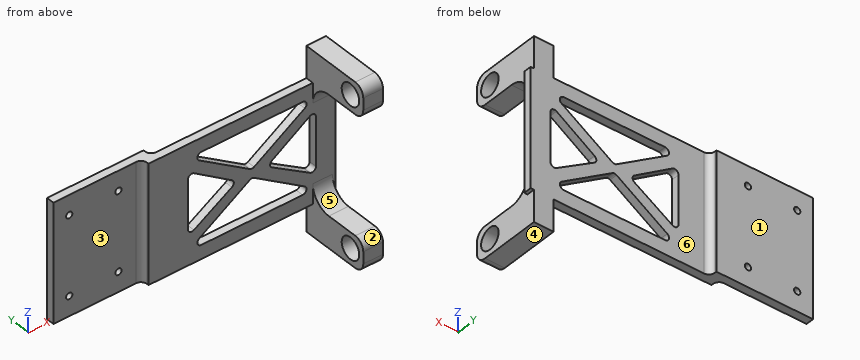
from build123d import *

# Parameters (mm, degrees)
BOSS_EXTRUDE1_DEPTH  = 60
FILLET1_R            = 3
CUT_EXTRUDE1_REACH   = 120.661
SKETCH2_R            = 1.6
CUT_EXTRUDE2_REACH   = 120.458
FILLET2_R            = 2
SKETCH5_W            = 10
SKETCH5_H            = 4
BOSS_EXTRUDE2_DEPTH  = 16
SKETCH6_W            = 10
SKETCH6_H            = 16
BOSS_EXTRUDE3_DEPTH  = 31.5
CUT_EXTRUDE3_REACH   = 163.612
SKETCH7_R            = 5.45
FILLET3_R            = 5
FILLET4_R            = 10
FILLET3_OF_MIRROR3_R = 5
FILLET4_OF_MIRROR3_R = 10


with BuildPart() as part:
    # Sketch1 → Boss-Extrude1 (new body)
    with BuildSketch(Plane.XY):
        Polygon((-37.939393939, 0.885392049), (7.060606061, 0.885392049), (7.060606061, -3.114607951), (102.060606061, -3.114607951), (102.060606061, 0.885392049), (11.060606061, 0.885392049), (11.060606061, 4.885392049), (-37.939393939, 4.885392049), align=None)
    extrude(amount=BOSS_EXTRUDE1_DEPTH)

    # Fillet1
    fillet1_edges = [part.edges().sort_by_distance(p)[0] for p in [
        (7.060606061, 0.885392049, 30),
        (11.060606061, 0.885392049, 30),
    ]]
    fillet(fillet1_edges, radius=FILLET1_R)

    # Sketch2 → Cut-Extrude1 (cut, up to next)
    with BuildSketch(Plane(origin=(0, 4.885392049, 0), x_dir=(1, 0, 0), z_dir=(0, 1, 0)), mode=Mode.PRIVATE) as cut_extrude1_sk1:
        with Locations(Location((-4.939393939, -50, 0), (0, 0, 180))):
            Circle(SKETCH2_R)
    cut_extrude1_tool1 = extrude(cut_extrude1_sk1.sketch, amount=-CUT_EXTRUDE1_REACH, mode=Mode.PRIVATE) & part.part
    # Sketch2 → Cut-Extrude1 (cut, up to next)
    with BuildSketch(Plane(origin=(0, 4.885392049, 0), x_dir=(1, 0, 0), z_dir=(0, 1, 0)), mode=Mode.PRIVATE) as cut_extrude1_sk2:
        with Locations(Location((-29.939393939, -50, 0), (0, 0, 180))):
            Circle(SKETCH2_R)
    cut_extrude1_tool2 = extrude(cut_extrude1_sk2.sketch, amount=-CUT_EXTRUDE1_REACH, mode=Mode.PRIVATE) & part.part
    cut_extrude1_1 = cut_extrude1_tool1.solids().sort_by_distance((-4.939394, 4.885392, 50))[0]
    add(cut_extrude1_1, mode=Mode.SUBTRACT)
    cut_extrude1_2 = cut_extrude1_tool2.solids().sort_by_distance((-29.939394, 4.885392, 50))[0]
    add(cut_extrude1_2, mode=Mode.SUBTRACT)
    cut_extrude1 = cut_extrude1_1 + cut_extrude1_2  # Cut-Extrude1 as one shape, for the pattern or mirror that repeats it

    # Mirror2: Cut-Extrude1 across plane
    add(cut_extrude1.mirror(Plane.XY.offset(30)), mode=Mode.SUBTRACT)

    # Sketch4 → Cut-Extrude2 (cut, up to next)
    with BuildSketch(Plane(origin=(0, 0.885392049, 0), x_dir=(1, 0, 0), z_dir=(0, 1, 0)), mode=Mode.PRIVATE) as cut_extrude2_sk1:
        Polygon((27.060606061, -14.276205352), (27.060606061, -46.276205352), (52.060606061, -29.743980797), align=None)
    cut_extrude2_tool1 = extrude(cut_extrude2_sk1.sketch, amount=-CUT_EXTRUDE2_REACH, mode=Mode.PRIVATE) & part.part
    # Sketch4 → Cut-Extrude2 (cut, up to next)
    with BuildSketch(Plane(origin=(0, 0.885392049, 0), x_dir=(1, 0, 0), z_dir=(0, 1, 0)), mode=Mode.PRIVATE) as cut_extrude2_sk2:
        Polygon((59.560606061, -32), (27.060606061, -53), (92.060606061, -53), align=None)
    cut_extrude2_tool2 = extrude(cut_extrude2_sk2.sketch, amount=-CUT_EXTRUDE2_REACH, mode=Mode.PRIVATE) & part.part
    # Sketch4 → Cut-Extrude2 (cut, up to next)
    with BuildSketch(Plane(origin=(0, 0.885392049, 0), x_dir=(1, 0, 0), z_dir=(0, 1, 0)), mode=Mode.PRIVATE) as cut_extrude2_sk3:
        Polygon((67.060606061, -29.743980797), (92.060606061, -14.276205352), (92.060606061, -46.276205352), align=None)
    cut_extrude2_tool3 = extrude(cut_extrude2_sk3.sketch, amount=-CUT_EXTRUDE2_REACH, mode=Mode.PRIVATE) & part.part
    # Sketch4 → Cut-Extrude2 (cut, up to next)
    with BuildSketch(Plane(origin=(0, 0.885392049, 0), x_dir=(1, 0, 0), z_dir=(0, 1, 0)), mode=Mode.PRIVATE) as cut_extrude2_sk4:
        Polygon((92.060606061, -7), (59.560606061, -28), (27.060606061, -7), align=None)
    cut_extrude2_tool4 = extrude(cut_extrude2_sk4.sketch, amount=-CUT_EXTRUDE2_REACH, mode=Mode.PRIVATE) & part.part
    add(cut_extrude2_tool1.solids().sort_by_distance((35.393939, 0.885392, 30.098797))[0], mode=Mode.SUBTRACT)
    add(cut_extrude2_tool2.solids().sort_by_distance((59.560606, 0.885392, 46))[0], mode=Mode.SUBTRACT)
    add(cut_extrude2_tool3.solids().sort_by_distance((83.727273, 0.885392, 30.098797))[0], mode=Mode.SUBTRACT)
    add(cut_extrude2_tool4.solids().sort_by_distance((59.560606, 0.885392, 14))[0], mode=Mode.SUBTRACT)

    # Fillet2
    fillet2_edges = [part.edges().sort_by_distance(p)[0] for p in [
        (59.560606061, -1.114607951, 32),
        (92.060606061, -1.114607951, 53),
        (27.060606061, -1.114607951, 53),
        (92.060606061, -1.114607951, 46.276205352),
        (67.060606061, -1.114607951, 29.743980797),
        (92.060606061, -1.114607951, 14.276205352),
        (27.060606061, -1.114607951, 7),
        (92.060606061, -1.114607951, 7),
        (59.560606061, -1.114607951, 28),
        (27.060606061, -1.114607951, 14.276205352),
        (52.060606061, -1.114607951, 29.743980797),
        (27.060606061, -1.114607951, 46.276205352),
    ]]
    fillet(fillet2_edges, radius=FILLET2_R)

    # Sketch5 → Boss-Extrude2 (add)
    with BuildSketch(Plane.XY.offset(60)):
        with Locations((95.422932692, -1.114607951)):
            Rectangle(SKETCH5_W, SKETCH5_H)
    boss_extrude2 = extrude(amount=BOSS_EXTRUDE2_DEPTH)

    # Sketch6 → Boss-Extrude3 (add)
    with BuildSketch(Plane.XZ.offset(3.114607951)):
        with Locations((95.422932692, 68)):
            Rectangle(SKETCH6_W, SKETCH6_H)
    boss_extrude3 = extrude(amount=BOSS_EXTRUDE3_DEPTH)

    # Sketch7 → Cut-Extrude3 (cut, up to next)
    with BuildSketch(Plane(origin=(100.422932692, 0, 0), x_dir=(0, 0, -1), z_dir=(1, 0, 0)), mode=Mode.PRIVATE) as cut_extrude3_sk1:
        with Locations((-68, -26.614607951)):
            Circle(SKETCH7_R)
    cut_extrude3_tool1 = extrude(cut_extrude3_sk1.sketch, amount=-CUT_EXTRUDE3_REACH, mode=Mode.PRIVATE) & part.part
    cut_extrude3 = cut_extrude3_tool1.solids().sort_by_distance((100.422933, -26.614608, 68))[0]
    add(cut_extrude3, mode=Mode.SUBTRACT)

    # Fillet3
    fillet3_edges = [part.edges().sort_by_distance(p)[0] for p in [
        (95.422932692, -34.614607951, 60),
        (95.422932692, -34.614607951, 76),
    ]]
    fillet(fillet3_edges, radius=FILLET3_R)

    # Fillet4
    fillet4_edges = [part.edges().sort_by_distance(p)[0] for p in [
        (95.422932692, -3.114607951, 60),
    ]]
    fillet(fillet4_edges, radius=FILLET4_R)

    # Mirror3: Boss-Extrude2, Boss-Extrude3, Cut-Extrude3 across plane
    add(boss_extrude2.mirror(Plane.XY.offset(30)))
    add(boss_extrude3.mirror(Plane.XY.offset(30)))
    add(cut_extrude3.mirror(Plane.XY.offset(30)), mode=Mode.SUBTRACT)

    # Fillet3 of Mirror3
    fillet3_of_mirror3_edges = [part.edges().sort_by_distance(p)[0] for p in [
        (95.422932692, -34.614607951, 0),
        (95.422932692, -34.614607951, -16),
    ]]
    fillet(fillet3_of_mirror3_edges, radius=FILLET3_OF_MIRROR3_R)

    # Fillet4 of Mirror3
    fillet4_of_mirror3_edges = [part.edges().sort_by_distance(p)[0] for p in [
        (95.422932692, -3.114607951, 0),
    ]]
    fillet(fillet4_of_mirror3_edges, radius=FILLET4_OF_MIRROR3_R)


solid = part.part
Geometry: final body of the model. Coordinates: model frame, mm. Face numbers are marked on the shaded views. A direction names the side the tool comes from. Round coordinates to 2 decimals unless told otherwise and drop trailing zeros. Order: outer loops, then holes, each group sorted by start corner. A loop starts at its lowest first (then second) coordinate and runs counter-clockwise, first axis right, second up. Notation, with made-up numbers: (-38.5, 71.5) -> (-34.5, 71.5) arc R28 cw to (-34.5, 97.5) -> close; hole circle Ø6 at (-15.5, 70). An arc over 180 degrees is marked (long way). Put each result on its own line as item: value. Start each with the question number.
Q1. Pull-direction query (Z, two-part tool) for the marked faces 4, 5 and 6; classes: +Z half, -Z half, draft (parallel to the pull), parting line (faces both ways), or undercut.
Q2. Section C-C on y = -7. Return the cut outline in (x, z).
Q3. First-contact query: pin 1 (3 mm diameter, centred on x = -4.94, z = 50, fed in from +Y); pin 2 (2 mm diameter, centred on x = 63.5, y = -1.5, fed in from +Z); pin 3 (12.5 mm diameter, centred on x = -24, z = 18.5, fed in from -Y); pin 4 (2 mm diameter, centred on x = 11.5, z = 14, fed in from +Y). Flat tips, straight axial feed; report the tip coordinate or a pass-through.
Q4. Section B-B on x = 54. Return the cut outline in (y, z), and give its area (3 significant figures).
Q5. Line query: probe 1 along X at (y, z) = (3.9, 10); probe 2 along Y at (x, z) = (28.5, 53.5); probe 3 along Z at (x, y) = (94.5, -12.5). Output: solid intervals per line, ascending.
Q6. Section A-A on z = 68. Return the cut outline in (x, y), and give its area (3 significant figures).
Q7. Reachability of the marked faces 1, 2 and 3 from +Z, -Z, +X, -X, +Y, -Y: full face, straight path, thin tool, end or side. Return the list, or none.
Ans:
1. face 4: -Z half
1. face 5: undercut
1. face 6: draft
2. outline: (90.42, -16) -> (100.42, -16) -> (100.42, 2.09) -> (90.42, 2.09) -> close; (90.42, 57.91) -> (100.42, 57.91) -> (100.42, 76) -> (90.42, 76) -> close
3. pin 1: passes through
3. pin 2: stops at z = 60
3. pin 3: stops at y = 0.89
3. pin 4: stops at y = 4.89
4. outline: (-3.11, 0) -> (0.89, 0) -> (0.89, 7) -> (-3.11, 7) -> close; (-3.11, 24.41) -> (0.89, 24.41) -> (0.89, 35.59) -> (-3.11, 35.59) -> close; (-3.11, 53) -> (0.89, 53) -> (0.89, 60) -> (-3.11, 60) -> close
4. area: 101 mm2
5. probe 1: x = -37.94 to -31.54, -28.34 to -6.54, -3.34 to 11.06
5. probe 2: y = -3.11 to 0.89
5. probe 3: z = -16 to 0.02, 59.98 to 76
6. outline: (90.42, -34.61) -> (100.42, -34.61) -> (100.42, -32.06) -> (90.42, -32.06) -> close; (90.42, -21.16) -> (100.42, -21.16) -> (100.42, 0.89) -> (90.42, 0.89) -> close
6. area: 246 mm2
7. face 1: +Z, -Z, +X, -X, +Y
7. face 2: +X, -X, -Y
7. face 3: +Z, -Z, -X, -Y
